```python
from build123d import *

# Parameters (mm, degrees)
F0_W     = 100
F0_H     = 100
F1_DEPTH = 90
F3_DEPTH = 100.001
F5_DEPTH = 100.001
F7_DEPTH = 100.001
F9_DEPTH = 100.001


with BuildPart() as f1:
    # F0 (on Top) → F1 (new body)
    with BuildSketch(Plane.XY):
        Rectangle(F0_W, F0_H)
    extrude(amount=F1_DEPTH)

    # F2 (on face) → F3 (cut, through all)
    with BuildSketch(Plane.YZ.offset(50)):
        Polygon((-20, 20), (-20, 0), (20, 0), (20, 20), (0, 6), align=None)
    extrude(amount=-F3_DEPTH, mode=Mode.SUBTRACT)

    # F4 (on face) → F5 (cut, through all)
    with BuildSketch(Plane.XZ.offset(50)):
        Polygon((-20, 20), (-20, 0), (20, 0), (20, 20), (0, 6), align=None)
    extrude(amount=-F5_DEPTH, mode=Mode.SUBTRACT)

    # F6 (on face) → F7 (cut, through all)
    with BuildSketch(Plane.YZ.offset(50)):
        Polygon((12, 90), (-12, 90), (0, 75), align=None)
    extrude(amount=-F7_DEPTH, mode=Mode.SUBTRACT)

    # F8 (on face) → F9 (cut, through all)
    with BuildSketch(Plane.XZ.offset(50)):
        Polygon((12, 90), (-12, 90), (0, 75), align=None)
    extrude(amount=-F9_DEPTH, mode=Mode.SUBTRACT)


solid = f1.part
```
Model file for the job. Use its own axes, mm. A direction names the side the tool comes from. Coordinates: 2 decimals unless noted, no trailing zeros. Loops run counter-clockwise (first coordinate to the right, second up) from the corner with the lowest first, then second, coordinate; pieces in that order, holes last. Notation, with made-up numbers: (47, 58) - (62, 58) arc R14 cw to (62, 83) - close; hole circle Ø6 at (-15.75, 8.5). An arc over 180 degrees is marked (long way). Answer as a JSON object with one key per item and string values. Group by question number.
(1) Flat gauge pins, fed straight in: pin 1 (5 mm diameter, centred on x = -12.5, y = 34, fed in from -Z); pin 2 (4 mm diameter, centred on x = -17.5, y = -39, fed in from -Z). Where does each tip first touch, or does it go through?
(2) Cut at B-B (y = 30.5). Give the cut face in (x, z), then the cut area to 3 significant figures.
(3) Tool access for faces 1 (the face through (-35, 20, 10)), 2 (the face through (-30.21, -6.08, 82.6)), 3 (the face through (-6.08, 30.21, 82.6)), 4 (the face through (10, -35, 13)): list every direction of +Z, -Z, +X, -X, +Y, -Y with a clear straight run to the whole face (end or side of a thin tool).
(4) Two-plate mould, pull along Y, no slides. Class faces 5 (the face through (31, -31, 90)), 6 (the face through (-35, -20, 10)): released by +Y, released by -Y, zero draft, split by the parting line, or undercut.
(5) Cut at D-D (y = 18.5). Give the cut face in (x, z), then the cut area to 3 significant figures.
(6) Probe line 1 along Y through (x, z) = (43, 7.5); line 2 along Y through (x, z) = (26, 82.5); line 3 along Z through (x, y) = (-16.5, 30). List the from-to ranges inside material, lowest first.
(7) Cut at C-C (x = -17). Give the cut face in (y, z), then the cut area to 3 significant figures.
(8) Cut at A-A (z = 76.5). Give the cut face in (x, y), then the cut area to 3 significant figures.
Geometry says:
{
 "1": {"pin 1": "stops at z = 13", "pin 2": "stops at z = 16.85"},
 "2": {"outline": "(-50, 0) - (-20, 0) - (-20, 20) - (0, 6) - (20, 20) - (20, 0) - (50, 0) - (50, 90) - (12, 90) - (0, 75) - (-12, 90) - (-50, 90) - close", "area": "8,300 mm^2"},
 "3": {"face 1": "-Z, +X, -X", "face 2": "+Z, +X, -X", "face 3": "+Z, +Y, -Y", "face 4": "-Z, +Y, -Y"},
 "4": {"face 5": "zero draft", "face 6": "undercut"},
 "5": {"outline": "(-50, 18.95) - (-20, 18.95) - (-20, 20) - (-18.5, 18.95) - (18.5, 18.95) - (20, 20) - (20, 18.95) - (50, 18.95) - (50, 90) - (12, 90) - (0, 75) - (-12, 90) - (-50, 90) - close", "area": "6,920 mm^2"},
 "6": {"line 1": "y = -50 to -20, -2.14 to 2.14, 20 to 50", "line 2": "y = -50 to -6, 6 to 50", "line 3": "z = 17.55 to 90"},
 "7": {"outline": "(-50, 17.9) - (-20, 17.9) - (-20, 20) - (-17, 17.9) - (17, 17.9) - (20, 20) - (20, 17.9) - (50, 17.9) - (50, 90) - (12, 90) - (0, 75) - (-12, 90) - (-50, 90) - close", "area": "7,020 mm^2"},
 "8": {"outline": "(-50, -50) - (-1.2, -50) - (-1.2, -1.2) - (-50, -1.2) - close; (-50, 1.2) - (-1.2, 1.2) - (-1.2, 50) - (-50, 50) - close; (1.2, -50) - (50, -50) - (50, -1.2) - (1.2, -1.2) - close; (1.2, 1.2) - (50, 1.2) - (50, 50) - (1.2, 50) - close", "area": "9,530 mm^2"}
}
